Check sheet for the modelled part. Datum: model origin and axes. Units: mm. A direction names the side the tool comes from. Coordinates: 2 decimals unless noted, no trailing zeros. Loops run counter-clockwise (first coordinate to the right, second up) from the corner with the lowest first, then second, coordinate; pieces in that order, holes last. Notation, with made-up numbers: (40, -2) -> (64, -2) arc R11 cw to (64, 3) -> close; hole circle Ø9 at (14, -7). An arc over 180 degrees is marked (long way). Use CSV: the item, a comma, the result in double quotes. Start each with the question number.
1. Sectioned sample at D-D, the plane y = -2. Record the cut outline in (x, z).
2. Sectioned sample at A-A, the plane y = -19. Record the cut outline in (x, z).
3. Release check for a two-part mould opening along X. For faces 1 (the face through (0, -4, 1.778)), 2 (the face through (31.191, -27, 2)), 3 (the face through (-27.435, -32.894, 2.712)), 4 (the face through (-21.816, -6.39, 1.159)) record: pulls with the +X half, pulls with the -X half, needs draft (parallel to the pull), parting line crosses it, or undercut.
4. Sectioned sample at B-B, the plane z = 3. Record the cut outline in (x, y) (3 decimals).
5. Set-up check for faces 5 (the face through (23.571, -19, 1)), 6 (the face through (-24.344, -29.959, 2.704)), 7 (the face through (-20.124, -8.96, 2.036)): record each of +Z, -Z, +X, -X, +Y, -Y from which the full face is reachable in a straight line by a thin tool's end or side.
6. Gauge pin test, flat ends, axial feed: pin 1 (0.9 mm diameter, centred on x = -1, z = 1, fed in from -Y); pin 2 (12.5 mm diameter, centred on x = -10.5, y = -6.5, fed in from +Z); pin 3 (3 mm diameter, centred on x = -27.38, y = -15.24, fed in from -Z); pin 4 (10.5 mm diameter, centred on x = -27.5, y = -12.5, fed in from +Z). Record the tip position at first contact, or that the pin passes through.
7. Sectioned sample at C-C, the plane x = -3. Record the cut outline in (y, z), and give its area (3 significant figures).
8. Thickness scan on L1, parallel to X at y = -29, z = 4.5; L2, parallel to X at y = -21, z = 0.6; L3, parallel to Z at x = -26.5, y = -23.5. Record the ranges inside material, lowest first.
```python
from build123d import *

# Parameters (mm, degrees)
BOSS_EXTRUDE1_DEPTH                  = 6.35
CUT_START                            = -8.62
SKETCH2_R                            = 1.0033
CUT_FOR_LID_MOUNT_SCREW_DEPTH        = 33.1912
SKETCH3_R                            = 1.8415
CUT_FOR_MOUNTING_SCREW_DEPTH         = 7.35
CUT_FOR_CONTROL_WIRE_CLEARANCE_DEPTH = 7.35
BOSS_EXTRUDE2_DEPTH                  = 6.35
CUT_EXTRUDE1_DEPTH                   = 7.35
CUT_EXTRUDE2_DEPTH                   = 63.3824
SKETCH18_W                           = 1.016
SKETCH18_H                           = 8.944323542
CUT_EXTRUDE11_DEPTH                  = 63.3824
CUT_EXTRUDE12_DEPTH                  = 0.508


with BuildPart() as part:
    # Sketch1 → Boss-Extrude1 (new body)
    with BuildSketch(Plane.XY):
        Polygon((0, 0), (-31.1912, 0), (-31.1912, -36.195), (-23.5712, -36.195), (-23.5712, -7.62), (0, -7.62), align=None)
    boss_extrude1 = extrude(amount=BOSS_EXTRUDE1_DEPTH)

    # Sketch2 → cut for lid mount screw (cut)
    with BuildSketch(Plane(origin=(-23.5712, 0, 0), x_dir=(0, 0, -1), z_dir=(1, 0, 0)).offset(CUT_START)):
        with Locations((-3.175, -32.004)):
            Circle(SKETCH2_R)
    cut_for_lid_mount_screw = extrude(amount=CUT_FOR_LID_MOUNT_SCREW_DEPTH, mode=Mode.SUBTRACT)

    # Sketch3 → cut for mounting screw (cut, through all)
    with BuildSketch(Plane.XY.offset(6.35)):
        with Locations((-27.3812, -15.24)):
            Circle(SKETCH3_R)
    cut_for_mounting_screw = extrude(amount=-CUT_FOR_MOUNTING_SCREW_DEPTH, mode=Mode.SUBTRACT)

    # Mirror1: Boss-Extrude1 across plane
    add(boss_extrude1.mirror(Plane(origin=(0, 0, 0), x_dir=(0, 0, 1), z_dir=(1, 0, 0))))

    # Mirror2: cut for lid mount screw across plane
    add(cut_for_lid_mount_screw.mirror(Plane(origin=(0, 0, 0), x_dir=(0, 0, 1), z_dir=(1, 0, 0))), mode=Mode.SUBTRACT)

    # Mirror3: cut for mounting screw across plane
    add(cut_for_mounting_screw.mirror(Plane(origin=(0, 0, 0), x_dir=(0, 0, 1), z_dir=(1, 0, 0))), mode=Mode.SUBTRACT)

    # Sketch4 → cut for control wire clearance (cut, through all)
    with BuildSketch(Plane.XY.offset(6.35)):
        Polygon((-25.0952, -24.384), (-25.0952, -29.207906516), (-23.5712, -30.731906516), (-23.5712, -22.86), align=None)
        Polygon((-23.5712, -36.195), (-23.5712, -33.655), (-26.1112, -36.195), align=None)
    cut_for_control_wire_clearance = extrude(amount=-CUT_FOR_CONTROL_WIRE_CLEARANCE_DEPTH, mode=Mode.SUBTRACT)

    # Mirror4: cut for control wire clearance across plane
    add(cut_for_control_wire_clearance.mirror(Plane(origin=(0, 0, 0), x_dir=(0, 0, 1), z_dir=(1, 0, 0))), mode=Mode.SUBTRACT)

    # Sketch5 → Boss-Extrude2 (add)
    with BuildSketch(Plane.XY.offset(6.35)):
        Polygon((-23.5712, -15.24), (-12.7, -7.62), (-13.297814932, 0), (-31.1912, -12.542092337), (-25.168706666, -12.542092337), align=None)
    boss_extrude2 = extrude(amount=-BOSS_EXTRUDE2_DEPTH)

    # Sketch6 → Cut-Extrude1 (cut, through all)
    with BuildSketch(Plane.XY.offset(6.35)):
        Polygon((-12.7, 0), (-31.1912, -12.961121495), (-31.1912, 0), align=None)
    cut_extrude1 = extrude(amount=-CUT_EXTRUDE1_DEPTH, mode=Mode.SUBTRACT)

    # Mirror5: Boss-Extrude2, Cut-Extrude1 across plane
    add(boss_extrude2.mirror(Plane(origin=(0, 0, 0), x_dir=(0, 0, 1), z_dir=(1, 0, 0))))
    add(cut_extrude1.mirror(Plane(origin=(0, 0, 0), x_dir=(0, 0, 1), z_dir=(1, 0, 0))), mode=Mode.SUBTRACT)

    # Sketch7 → Cut-Extrude2 (cut, through all)
    with BuildSketch(Plane.ZY.offset(31.1912)):
        Polygon((6.35, -28.575), (4.201541935, -28.012372807), (2.286, -26.197127086), (2.286, -0.156208848), (0, 0), (6.35, 0), align=None)
        Polygon((0, -36.195), (6.35, -36.195), (6.35, -35.639446987), align=None)
    extrude(amount=-CUT_EXTRUDE2_DEPTH, mode=Mode.SUBTRACT)

    # Sketch18 → Cut-Extrude11 (cut, through all)
    with BuildSketch(Plane(origin=(31.1912, 0, 0), x_dir=(0, 0, -1), z_dir=(1, 0, 0))):
        with Locations((-5.842, -31.986995599)):
            Rectangle(SKETCH18_W, SKETCH18_H)
    extrude(amount=-CUT_EXTRUDE11_DEPTH, mode=Mode.SUBTRACT)

    # Sketch19 → Cut-Extrude12 (cut)
    with BuildSketch(Plane.XY.offset(2.286)):
        Polygon((-22.057028978, -6.558665171), (-18.1356, -11.43), (-12.7, -7.62), (0, -7.62), (0, 0), (-12.7, 0), align=None)
    cut_extrude12 = extrude(amount=-CUT_EXTRUDE12_DEPTH, mode=Mode.SUBTRACT)

    # Mirror6: Cut-Extrude12 across plane
    add(cut_extrude12.mirror(Plane(origin=(0, 0, 0), x_dir=(0, 0, 1), z_dir=(1, 0, 0))), mode=Mode.SUBTRACT)


solid = part.part
```
Completed:
1,outline,"(-15.55, 0) -> (15.55, 0) -> (15.55, 1.78) -> (-15.55, 1.78) -> close"
2,outline,"(-31.19, 0) -> (-23.57, 0) -> (-23.57, 2.29) -> (-31.19, 2.29) -> close; (23.57, 0) -> (31.19, 0) -> (31.19, 2.29) -> (23.57, 2.29) -> close"
3,face 1,"undercut"
3,face 2,"pulls with the +X half"
3,face 3,"needs draft"
3,face 4,"pulls with the -X half"
4,outline,"(-31.191, -35.933) -> (-25.849, -35.933) -> (-23.571, -33.655) -> (-23.571, -32.992) -> (-31.191, -32.992) -> close; (-31.191, -31.016) -> (-23.571, -31.016) -> (-23.571, -30.732) -> (-25.095, -29.208) -> (-25.095, -26.874) -> (-31.191, -26.874) -> close; (23.571, -33.655) -> (25.849, -35.933) -> (31.191, -35.933) -> (31.191, -32.992) -> (23.571, -32.992) -> close; (23.571, -31.016) -> (31.191, -31.016) -> (31.191, -26.874) -> (25.095, -26.874) -> (25.095, -29.208) -> (23.571, -30.732) -> close"
5,face 5,"+Z, -Z, -Y"
5,face 6,"+Z, -Z"
5,face 7,"+Z, +Y"
6,pin 1,"y = -7.62"
6,pin 2,"z = 1.78"
6,pin 3,"through"
6,pin 4,"z = 2.29"
7,outline,"(-7.62, 0) -> (0, 0) -> (-0.12, 1.78) -> (-7.62, 1.78) -> close"
7,area,"13.4 mm²"
8,L1,"-31.19 to -25.1, 25.1 to 31.19"
8,L2,"-31.19 to -23.57, 23.57 to 31.19"
8,L3,"0 to 2.29"
